For this review, take the finished solid that the model builds, in its own axes (mm). Face numbers are marked on the shaded views. A direction names the side the tool comes from. Give positions to 0.01 mm unless a question says otherwise; leave off trailing zeros. Order: outer loops, then holes, each group sorted by start corner. A loop starts at its lowest first (then second) coordinate and runs counter-clockwise, first axis right, second up. Notation, with made-up numbers: M 54,19 L 88,19 A25 cw 88,48 Z; hole C 83,7 d9. An arc over 180 degrees is marked long. Use CSV: the item, a comma, the result in double quotes. Start each with the question number.
(1) Draft analysis for pull direction X (two halves, no side actions). For the marked faces 6 and 7, state which applies: pulls with the +X half, pulls with the -X half, needs draft (parallel to the pull), parting line crosses it, or undercut.
(2) Tool access review of the marked faces 1, 2, 3, 4 and 5: name each direction out of +Z, -Z, +X, -X, +Y, -Y from which nothing blocks a thin tool from reaching the whole face with its end or side.
(3) Consider section A-A (z = -4.5). Write out the cut boundary in (x, y), and give its area (3 significant figures).
(4) Consider section C-C (y = 0). Give the number of separate pieces and of enclosed holes in the cut face, and give its area (3 significant figures).
(5) Wall thickness on L1, parallel to Y at x = 0, z = -19.1; L2, parallel to Y at x = 0, z = -23; L3, parallel to Z at x = 166.5, y = -26.5: over which ranges is each line inside the solid? List them lowest first. Write a range as from..to.
(6) Consider section B-B (x = 35). Write out the cut boundary in (y, z).
(7) Consider section D-D (x = 98.5). Write out the cut boundary in (y, z), and give its area (3 significant figures).
(8) Clearance check with flat-ended pins moving along their axes: P1, Ø10, axis at y = 6.5, z = -3.5, coming from the -X side; P2, Ø6, axis at y = -6, z = 3, coming from the -X side; P3, Ø10, axis at y = 26.5, z = 3.5, coming from the +X side; P4, Ø7, axis at x = 162, y = 34, coming from the -Z side. State where each tip first meets the part, or that it passes through.
```python
from build123d import *
from build123d.topology import SkipClean

# Parameters (mm, degrees)
SKETCH1_R           = 2
BOSS_EXTRUDE1_DEPTH = 25
SKETCH2_R           = 3
CUT_EXTRUDE2_DEPTH  = 5
CUT_EXTRUDE3_DEPTH  = 162.5
BOSS_EXTRUDE2_START = 20
SKETCH6_R           = 40
SKETCH6_R_2         = 38
BOSS_EXTRUDE2_DEPTH = 20
FILLET1_R           = 5


with BuildPart() as part:
    # Sketch1 → Boss-Extrude1 (new, symmetric)
    with BuildSketch(Plane.XY):
        with BuildLine():
            Line((80, -40), (0, -40))
            ThreePointArc((0, -40), (-40, 0), (0, 40))
            Line((0, 40), (80, 40))
            Line((80, 40), (82, 40))
            Line((82, 40), (162, 40))
            ThreePointArc((162, 40), (202, 0), (162, -40))
            Line((162, -40), (82, -40))
            Line((82, -40), (80, -40))
        make_face()
        with Locations((0, 34)):
            Circle(SKETCH1_R, mode=Mode.SUBTRACT)
        with Locations((29.444863729, 17)):
            Circle(SKETCH1_R, mode=Mode.SUBTRACT)
        with Locations((29.444863729, -17)):
            Circle(SKETCH1_R, mode=Mode.SUBTRACT)
        with Locations((0, -34)):
            Circle(SKETCH1_R, mode=Mode.SUBTRACT)
        with Locations((-29.444863729, -17)):
            Circle(SKETCH1_R, mode=Mode.SUBTRACT)
        with Locations((-29.444863729, 17)):
            Circle(SKETCH1_R, mode=Mode.SUBTRACT)
        with Locations(Location((162, -34, 0), (0, 0, 180))):
            Circle(SKETCH1_R, mode=Mode.SUBTRACT)
        with Locations(Location((191.444863729, 17, 0), (0, 0, 180))):
            Circle(SKETCH1_R, mode=Mode.SUBTRACT)
        with Locations(Location((191.444863729, -17, 0), (0, 0, 180))):
            Circle(SKETCH1_R, mode=Mode.SUBTRACT)
        with Locations(Location((132.555136271, -17, 0), (0, 0, 180))):
            Circle(SKETCH1_R, mode=Mode.SUBTRACT)
        with Locations(Location((132.555136271, 17, 0), (0, 0, 180))):
            Circle(SKETCH1_R, mode=Mode.SUBTRACT)
        with Locations(Location((162, 34, 0), (0, 0, 180))):
            Circle(SKETCH1_R, mode=Mode.SUBTRACT)
        with BuildLine():
            ThreePointArc((25, 0), (0, 25), (-25, 0))
            ThreePointArc((-25, 0), (0, -25), (25, 0))
        make_face(mode=Mode.SUBTRACT)
        with BuildLine():
            ThreePointArc((187, 0), (162, -25), (137, 0))
            ThreePointArc((137, 0), (162, 25), (187, 0))
        make_face(mode=Mode.SUBTRACT)
    extrude(amount=BOSS_EXTRUDE1_DEPTH, both=True)

    # Sketch2 → Cut-Extrude2 (cut)
    with BuildSketch(Plane(origin=(0, 0, -25), x_dir=(-1, 0, 0), z_dir=(0, 0, -1))):
        with Locations((-162, 34)):
            Circle(SKETCH2_R)
        with Locations((-132.555136271, 17)):
            Circle(SKETCH2_R)
        with Locations((-132.555136271, -17)):
            Circle(SKETCH2_R)
        with Locations((-162, -34)):
            Circle(SKETCH2_R)
        with Locations((-191.444863729, -17)):
            Circle(SKETCH2_R)
        with Locations((-191.444863729, 17)):
            Circle(SKETCH2_R)
        with Locations(Location((29.444863729, 17, 0), (0, 0, 180))):
            Circle(SKETCH2_R)
        with Locations(Location((29.444863729, -17, 0), (0, 0, 180))):
            Circle(SKETCH2_R)
        with Locations(Location((0, -34, 0), (0, 0, 180))):
            Circle(SKETCH2_R)
        with Locations(Location((-29.444863729, -17, 0), (0, 0, 180))):
            Circle(SKETCH2_R)
        with Locations(Location((-29.444863729, 17, 0), (0, 0, 180))):
            Circle(SKETCH2_R)
        with Locations(Location((0, 34, 0), (0, 0, 180))):
            Circle(SKETCH2_R)
    extrude(amount=-CUT_EXTRUDE2_DEPTH, mode=Mode.SUBTRACT)

    # Sketch5 → Cut-Extrude3 (cut, symmetric)
    with BuildSketch(Plane(origin=(0, 0, 0), x_dir=(1, 0, 0), z_dir=(0, 1, 0))):
        Polygon((61, -0.703195853), (61, -5), (101, -5), (101, -0.703195853), (105.532166919, 25), (56.467833081, 25), align=None)
        Polygon((54.75, -1.25), (51.223460386, 18.75), (-40, 18.75), (-40, -25), (202, -25), (202, 18.75), (110.776539614, 18.75), (107.25, -1.25), (107.25, -11.25), (54.75, -11.25), align=None)
    extrude(amount=CUT_EXTRUDE3_DEPTH, both=True, mode=Mode.SUBTRACT)

    # Sketch6 → Boss-Extrude2 (add)
    # profile 1 of 2: a face of its own
    with SkipClean():  # the faces are left unmerged after this step: merging them gives an invalid solid
        with BuildSketch(Plane.XY.offset(-18.75).offset(BOSS_EXTRUDE2_START)):
            with Locations(Location((0, 0, 0), (0, 0, 270))):
                Circle(SKETCH6_R)
            Circle(SKETCH6_R_2, mode=Mode.SUBTRACT)
        # profile 2 of 2: a face of its own
        with BuildSketch(Plane.XY.offset(-18.75).offset(BOSS_EXTRUDE2_START)):
            with Locations(Location((162, 0, 0), (0, 0, 180))):
                Circle(SKETCH6_R)
            with Locations(Location((162, 0, 0), (0, 0, 180))):
                Circle(SKETCH6_R_2, mode=Mode.SUBTRACT)
        extrude(amount=-BOSS_EXTRUDE2_DEPTH)

    # Fillet1
    fillet1_edges = [part.edges().sort_by_distance(p)[0] for p in [
        (54.75, 0, 11.25),
        (107.25, 0, 11.25),
        (61, 0, 0.703195853),
        (101, 0, 0.703195853),
    ]]
    fillet(fillet1_edges, radius=FILLET1_R)


solid = part.part
```
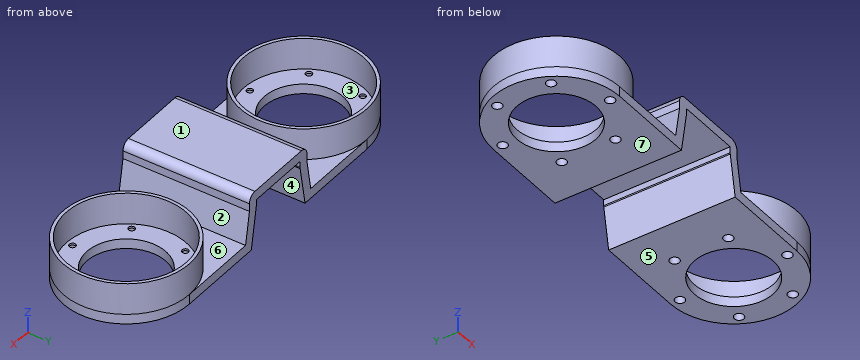
Check result:
1,face 6,"undercut"
1,face 7,"needs draft"
2,face 1,"+Z, +X, -X, +Y, -Y"
2,face 2,"+Z, +Y, -Y"
2,face 3,"+Z"
2,face 4,"-Z, +Y, -Y"
2,face 5,"-Z, +X, -X, +Y, -Y"
3,outline,"C 0,0 d80; M 53.74,-40 L 60.08,-40 L 60.08,40 L 53.74,40 Z; M 101.92,-40 L 108.26,-40 L 108.26,40 L 101.92,40 Z; C 162,0 d80; hole C 0,0 d76; hole C 162,0 d76"
3,area,"2,000 mm^2"
4,separate pieces,"3"
4,enclosed holes,"0"
4,area,"1,370 mm^2"
5,L1,"y = -40..-36, -32..-25, 25..32, 36..40"
5,L2,"y = -40..-37, -31..-25, 25..31, 37..40"
5,L3,"z = -25..-18.75"
6,outline,"M -40,-25 L 40,-25 L 40,-18.75 L 19.36,-18.75 L 19.36,1.25 L 14.8,1.25 L 14.8,-18.75 L -14.8,-18.75 L -14.8,1.25 L -19.36,1.25 L -19.36,-18.75 L -40,-18.75 Z"
7,outline,"M -40,5 L 40,5 L 40,11.25 L -40,11.25 Z"
7,area,"500 mm^2"
8,P1,"stops at x = -39.97"
8,P2,"stops at x = -39.84"
8,P3,"stops at x = 195.38"
8,P4,"stops at z = -25"
